Build history of the part. All positions in model axes, mm. Face numbers are marked on the shaded views. A direction names the side the tool comes from. Coordinates: 2 decimals unless noted, no trailing zeros. Order: outer loops, then holes, each group sorted by start corner. A loop starts at its lowest first (then second) coordinate and runs counter-clockwise, first axis right, second up. Notation, with made-up numbers: (48, 68.5) - (59, 68.5) arc R27 cw to (59, 97.5) - close; hole circle Ø2 at (25.25, 3.25). An arc over 180 degrees is marked (long way). Answer as CSV lines item,"result". Start each with the question number.
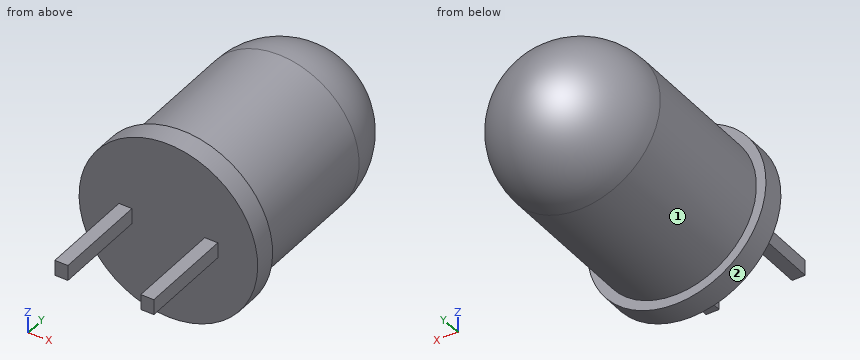
from build123d import *

# Parameters (mm, degrees)
SKETCH2_R           = 2.5
BOSS_EXTRUDE1_DEPTH = 7
SKETCH3_R           = 2.8
BOSS_EXTRUDE2_DEPTH = 0.7
FILLET1_R           = 2.5
SKETCH4_W           = 0.409361502
SKETCH4_H           = 0.4847702
BOSS_EXTRUDE3_DEPTH = 3


with BuildPart() as part:
    # Sketch2 → Boss-Extrude1 (new body)
    with BuildSketch(Plane(origin=(0, 0, 0), x_dir=(1, 0, 0), z_dir=(0, 1, 0))):
        with Locations(Location((0, 0, 0), (0, 0, 270))):
            Circle(SKETCH2_R)
    extrude(amount=BOSS_EXTRUDE1_DEPTH)

    # Sketch3 → Boss-Extrude2 (add)
    with BuildSketch(Plane.XZ):
        with Locations(Location((0, 0, 0), (0, 0, 270))):
            Circle(SKETCH3_R)
    extrude(amount=BOSS_EXTRUDE2_DEPTH)

    # Fillet1
    fillet1_edges = [part.edges().sort_by_distance(p)[0] for p in [
        (0, 7, -2.5),
    ]]
    fillet(fillet1_edges, radius=FILLET1_R)

    # Sketch4 → Boss-Extrude3 (add)
    with BuildSketch(Plane.XZ.offset(0.7)):
        with Locations((1.346583888, 0)):
            Rectangle(SKETCH4_W, SKETCH4_H)
        with Locations((-1.346583888, 0)):
            Rectangle(SKETCH4_W, SKETCH4_H)
    extrude(amount=BOSS_EXTRUDE3_DEPTH)


solid = part.part
(1) Drop flat-ended pins along their axis: pin 1 Ø0.5 at (x, y) = (1.5, -2.5) entering from +Z; pin 2 Ø3 at (x, z) = (0.5, -0.5) entering from -Y; pin 3 Ø1.5 at (y, z) = (-0.5, 1) entering from -X; pin 4 Ø0.5 at (y, z) = (-2, 0) entering from +X. Give the stop position or say it passes through.
(2) Band-saw the part on C-C on y = 0.5. List the corners of the cut face in (x, z), plus the area to 3 significant figures.
(3) Probe L1, parallel to Z at x = -0.05, y = 4.25; L2, parallel to Z at x = 1.2, y = -1.5; L3, parallel to Y at x = -1.95, z = -0.75. List the from-to ranges inside material, lowest first. Write a range as [from, to].
(4) Band-saw the part on D-D on x = 2.1. List the corners of the cut face in (y, z), plus the area to 3 significant figures.
(5) Which spindle directions (+Z, -Z, +X, -X, +Y, -Y) get a long thin tool onto all of the face, cutting with end or side? Do the marked faces 1 and 2. Say none if no direction does.
(6) Band-saw the part on A-A on x = 0. List the corners of the cut face in (y, z).
(7) Band-saw the part on B-B on z = 0. List the corners of the cut face in (x, y).
Filled in:
1,pin 1,"stops at z = 0.24"
1,pin 2,"stops at y = -3.7"
1,pin 3,"stops at x = -2.79"
1,pin 4,"stops at x = 1.55"
2,outline,"circle Ø5 at (0, 0)"
2,area,"19.6 mm^2"
3,L1,"z = [-2.5, 2.5]"
3,L2,"z = [-0.24, 0.24]"
3,L3,"y = [-0.7, 5.87]"
4,outline,"(-0.7, -1.85) - (0, -1.85) - (0, -1.36) - (4.5, -1.36) arc R1.36 ccw to (4.5, 1.36) - (0, 1.36) - (0, 1.85) - (-0.7, 1.85) - close"
4,area,"17.7 mm^2"
5,face 1,"+Y"
5,face 2,"+Y, -Y"
6,outline,"(-0.7, -2.8) - (0, -2.8) - (0, -2.5) - (4.5, -2.5) arc R2.5 ccw to (4.5, 2.5) - (0, 2.5) - (0, 2.8) - (-0.7, 2.8) - close"
7,outline,"(-2.8, -0.7) - (-1.55, -0.7) - (-1.55, -3.7) - (-1.14, -3.7) - (-1.14, -0.7) - (1.14, -0.7) - (1.14, -3.7) - (1.55, -3.7) - (1.55, -0.7) - (2.8, -0.7) - (2.8, 0) - (2.5, 0) - (2.5, 4.5) arc R2.5 ccw to (-2.5, 4.5) - (-2.5, 0) - (-2.8, 0) - close"
